Work out the finished part from the listing and answer in its coordinate system (mm). Face numbers are marked on the shaded views. A direction names the side the tool comes from. Round coordinates to 2 decimals unless told otherwise and drop trailing zeros. Order: outer loops, then holes, each group sorted by start corner. A loop starts at its lowest first (then second) coordinate and runs counter-clockwise, first axis right, second up. Notation, with made-up numbers: (28, -18) - (61, -18) arc R25 ccw to (61, 4) - close; hole circle Ø2 at (62.25, 43). An arc over 180 degrees is marked (long way). One line per question, with ' | ' between items. Start each with the question number.
from build123d import *

# Parameters (mm, degrees)
SKETCH_1_W          = 30
SKETCH_1_H          = 43
SKETCH_1_R          = 1.6
SKETCH_1_R_2        = 4
EXTRUDE_1_DEPTH     = 4
EXTRUDE_START       = -4
SKETCH_2_R          = 4
EXTRUDE_2_DEPTH     = 10
SKETCH_3_R          = 1.6
CUT_EXTRUDE_1_DEPTH = 11


with BuildPart() as part:
    # 草图1 → 凸台-拉伸1 (new body)
    with BuildSketch(Plane.XY):
        with Locations((-15, 24.658548848)):
            Rectangle(SKETCH_1_W, SKETCH_1_H)
        with Locations((-5, 8.158548848)):
            Circle(SKETCH_1_R, mode=Mode.SUBTRACT)
        with Locations((-25, 8.158548848)):
            Circle(SKETCH_1_R, mode=Mode.SUBTRACT)
        with Locations((-15, 38.158548848)):
            Circle(SKETCH_1_R_2, mode=Mode.SUBTRACT)
    extrude(amount=EXTRUDE_1_DEPTH)

    # 草图2 → 凸台-拉伸2 (add)
    with BuildSketch(Plane.XY.offset(4).offset(EXTRUDE_START)):
        with Locations((-15, 38.158548848)):
            Circle(SKETCH_2_R)
    extrude(amount=EXTRUDE_2_DEPTH)

    # 草图3 → 切除-拉伸1 (cut, through all)
    with BuildSketch(Plane.XY.offset(10)):
        with Locations((-15, 38.158548848)):
            Circle(SKETCH_3_R)
    extrude(amount=-CUT_EXTRUDE_1_DEPTH, mode=Mode.SUBTRACT)


solid = part.part
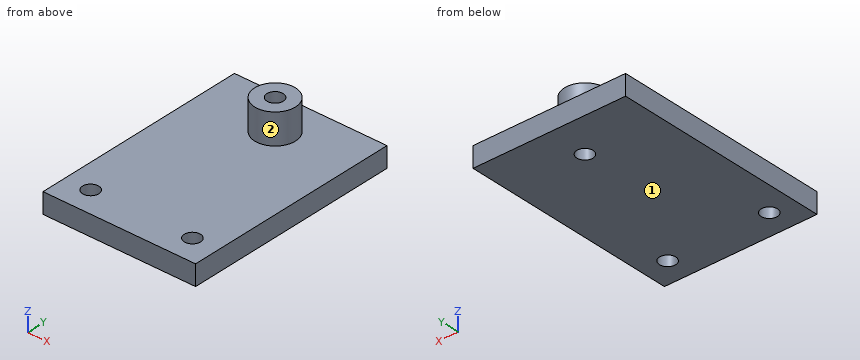
1) Section B-B on z = 2.75 is taken. Give the vertices of the cut face in (x, y).
2) Straight lines are drawn through the part: line 1 (Y direction, x = -15, z = 7.25); line 2 (Y direction, x = -5, z = 2.2); line 3 (Z direction, x = -9.75, y = 31). For each, find the intervals that lie inside material, in ascending order.
3) Section D-D on y = 41 is taken. Give the vertices of the cut face in (x, z).
4) Section C-C on x = -15 is taken. Give the vertices of the cut face in (y, z).
5) Flat-ended cylindrical pins translate along their axes: pin 1 (12 mm diameter, centred on x = -20.5, y = 13.5, fed in from +Z); pin 2 (2 mm diameter, centred on x = -12.5, z = 8, fed in from +Y); pin 3 (2.5 mm diameter, centred on x = -25, y = 8.16, fed in from -Z). Find the tip coordinate at first contact, or state that the pin passes through.
6) For the marked faces 1 and 2, determine the directions among +Z, -Z, +X, -X, +Y, -Y from which every point of the face is accessible in a straight line to the end or side of a thin tool.
7) Section A-A on x = -5 is taken. Give the vertices of the cut face in (y, z).
Recorded:
1) outline: (-30, 3.16) - (0, 3.16) - (0, 46.16) - (-30, 46.16) - close; hole circle Ø3.2 at (-25, 8.16); hole circle Ø3.2 at (-15, 38.16); hole circle Ø3.2 at (-5, 8.16)
2) line 1: y = 34.16 to 36.56, 39.76 to 42.16 | line 2: y = 3.16 to 6.56, 9.76 to 46.16 | line 3: z = 0 to 4
3) outline: (-30, 0) - (0, 0) - (0, 4) - (-12.18, 4) - (-12.18, 10) - (-17.82, 10) - (-17.82, 4) - (-30, 4) - close
4) outline: (3.16, 0) - (36.56, 0) - (36.56, 10) - (34.16, 10) - (34.16, 4) - (3.16, 4) - close; (39.76, 0) - (46.16, 0) - (46.16, 4) - (42.16, 4) - (42.16, 10) - (39.76, 10) - close
5) pin 1: stops at z = 4 | pin 2: stops at y = 41.87 | pin 3: passes through
6) face 1: -Z, +X, -X, +Y, -Y | face 2: +Z
7) outline: (3.16, 0) - (6.56, 0) - (6.56, 4) - (3.16, 4) - close; (9.76, 0) - (46.16, 0) - (46.16, 4) - (9.76, 4) - close
